from build123d import *

# Parameters (mm, degrees)
BOSS_EXTRUDE1_DEPTH = 1
CUT_EXTRUDE1_DEPTH  = 2


with BuildPart() as part:
    # Sketch1 → Boss-Extrude1 (new body)
    with BuildSketch(Plane.XY):
        with BuildLine():
            ThreePointArc((-10.45388601, -17.982109645), (0, -20.8), (10.45388601, -17.982109645))
            ThreePointArc((10.45388601, -17.982109645), (10.996786753, -15.931436881), (8.94611399, -15.388536138))
            ThreePointArc((8.94611399, -15.388536138), (0, -17.8), (-8.94611399, -15.388536138))
            ThreePointArc((-8.94611399, -15.388536138), (-10.996786753, -15.931436881), (-10.45388601, -17.982109645))
        make_face()
    extrude(amount=-BOSS_EXTRUDE1_DEPTH)

    # Sketch2 → Cut-Extrude1 (cut, through all)
    with BuildSketch(Plane.XY):
        with BuildLine():
            Line((-7.3, -17.853571071), (-7.3, -16.23422311))
            ThreePointArc((-7.3, -16.23422311), (-6.507590932, -16.567777771), (-5.7, -16.862680688))
            Line((-5.7, -16.862680688), (-5.7, -17.853571071))
            ThreePointArc((-5.7, -17.853571071), (-6.5, -18.653571071), (-7.3, -17.853571071))
        make_face()
        with BuildLine():
            Line((5.7, -17.853571071), (5.7, -16.862680688))
            ThreePointArc((5.7, -16.862680688), (6.507590932, -16.567777771), (7.3, -16.23422311))
            Line((7.3, -16.23422311), (7.3, -17.853571071))
            ThreePointArc((7.3, -17.853571071), (6.5, -18.653571071), (5.7, -17.853571071))
        make_face()
    extrude(amount=-CUT_EXTRUDE1_DEPTH, mode=Mode.SUBTRACT)


solid = part.part
Source: CAD feature listing. Evaluate the final solid. Frame: model axes, mm. A direction names the side the tool comes from. Coordinates: 2 decimals unless noted, no trailing zeros. Order: outer loops, then holes, each group sorted by start corner. A loop starts at its lowest first (then second) coordinate and runs counter-clockwise, first axis right, second up. Notation, with made-up numbers: M 60,11.5 L 119,11.5 A13 ccw 119,20.5 Z; hole C 77.5,86.25 d8. An arc over 180 degrees is marked long. Write each question's results on one line, items separated by ' | '. Start each with the question number.
Item 1: Draft query along X for faces 3 (the face through (7.3, -17, -0.5)), 4 (the face through (-0.2, -20.8, -0.5)), 5 (the face through (0, -18, 0)). Return one class per face: pulls with the +X half, pulls with the -X half, needs draft (parallel to the pull), parting line crosses it, or undercut.
Item 2: Cut plane C-C (x = 4). Return loops of the section in (y, z), and give its area (3 significant figures).
Item 3: Cut plane D-D (y = -20.1). Return loops of the section in (x, z), and give its area (3 significant figures).
Item 4: First-contact query: pin 1 Ø0.5 at (y, z) = (-17.5, -0.5) entering from -X. Flat tip, straight axial feed; report the tip coordinate or a pass-through.
Item 5: Cut plane B-B (z = -0.75). Return loops of the section in (x, y).
Item 6: Set-up query: faces 1 (the face through (0, -18, -1)), 2 (the face through (-8.12, -15.84, -0.49)). Return all of +Z, -Z, +X, -X, +Y, -Y with unobstructed straight access to the full face (end or side cutting, diameter ignored); none if empty.
Item 7: Cut plane A-A (y = -17.05). Return loops of the section in (x, z) (3 decimals), and give its area (4 significant figures).
Item 8: Line query: probe 1 along X at (y, z) = (-16.6, -0.2); probe 2 along X at (y, z) = (-18, -0.7); probe 3 along X at (y, z) = (-15.35, -0.2). Output: solid intervals per line, ascending.
Checked values:
1) face 3: undercut | face 4: parting line crosses it | face 5: needs draft
2) outline: M -20.41,-1 L -17.34,-1 L -17.34,0 L -20.41,0 Z | area: 3.07 mm2
3) outline: M -5.35,-1 L 5.35,-1 L 5.35,0 L -5.35,0 Z | area: 10.7 mm2
4) pin 1: stops at x = -11.09
5) outline: M -10.45,-17.98 A20.8 ccw 10.45,-17.98 A1.5 ccw 8.95,-15.39 A17.8 cw 7.3,-16.23 L 7.3,-17.85 A0.8 cw 5.7,-17.85 L 5.7,-16.86 A17.8 cw -5.7,-16.86 L -5.7,-17.85 A0.8 cw -7.3,-17.85 L -7.3,-16.23 A17.8 cw -8.95,-15.39 A1.5 ccw Z
6) face 1: -Z, +X, -X, +Y, -Y | face 2: +Z, -Z, +Y
7) outline: M -11.155,-1 L -7.3,-1 L -7.3,0 L -11.155,0 Z; M -5.7,-1 L -5.112,-1 L -5.112,0 L -5.7,0 Z; M 5.112,-1 L 5.7,-1 L 5.7,0 L 5.112,0 Z; M 7.3,-1 L 11.155,-1 L 11.155,0 L 7.3,0 Z | area: 8.885 mm2
8) probe 1: x = -11.2 to -7.3, 7.3 to 11.2 | probe 2: x = -10.42 to -7.29, -5.71 to 5.71, 7.29 to 10.42 | probe 3: x = -10.38 to -9.02, 9.02 to 10.38
